Input: part model. Units: mm. Frame: model coordinates. A direction names the side the tool comes from. Give positions to 0.01 mm unless a question says otherwise; leave off trailing zeros. Loops run counter-clockwise (first coordinate to the right, second up) from the corner with the lowest first, then second, coordinate; pieces in that order, holes last.
from build123d import *

# Parameters (mm, degrees)
SKETCH1_W           = 22
SKETCH1_H           = 4.5
BOSS_EXTRUDE1_DEPTH = 1
SKETCH2_W           = 4.5
SKETCH2_H           = 4.5
BOSS_EXTRUDE2_DEPTH = 5
FILLET1_R           = 0.5


with BuildPart() as part:
    # Sketch1 → Boss-Extrude1 (new body)
    with BuildSketch(Plane(origin=(0, 0, 0), x_dir=(1, 0, 0), z_dir=(0, 1, 0))):
        Rectangle(SKETCH1_W, SKETCH1_H)
    extrude(amount=BOSS_EXTRUDE1_DEPTH)

    # Sketch2 → Boss-Extrude2 (add)
    with BuildSketch(Plane(origin=(0, 1, 0), x_dir=(1, 0, 0), z_dir=(0, 1, 0))):
        with Locations((-8.75, 0)):
            Rectangle(SKETCH2_W, SKETCH2_H)
        with Locations((8.75, 0)):
            Rectangle(SKETCH2_W, SKETCH2_H)
    extrude(amount=BOSS_EXTRUDE2_DEPTH)

    # Fillet1
    fillet1_edges = [part.edges().sort_by_distance(p)[0] for p in [
        (8.75, 6, -2.25),
        (11, 6, 0),
        (8.75, 6, 2.25),
        (6.5, 6, 0),
        (-6.5, 6, 0),
        (-8.75, 6, 2.25),
        (-11, 6, 0),
        (-8.75, 6, -2.25),
    ]]
    fillet(fillet1_edges, radius=FILLET1_R)


solid = part.part
(1) Cut plane A-A (y = 2.15). Return the cut outline in (x, z).
Values follow:
outline: (-11, -2.25) - (-6.5, -2.25) - (-6.5, 2.25) - (-11, 2.25) - close; (6.5, -2.25) - (11, -2.25) - (11, 2.25) - (6.5, 2.25) - close
(2) Cut plane B-B (z = 0.65). Return the cut outline in (x, y), and give its area (3 significant figures).
Values follow:
outline: (-11, 0) - (11, 0) - (11, 5.5) arc R0.5 ccw to (10.5, 6) - (7, 6) arc R0.5 ccw to (6.5, 5.5) - (6.5, 1) - (-6.5, 1) - (-6.5, 5.5) arc R0.5 ccw to (-7, 6) - (-10.5, 6) arc R0.5 ccw to (-11, 5.5) - close
area: 66.8 mm2
(3) Cut plane C-C (x = -5.5). Return the cut outline in (y, z).
Values follow:
outline: (0, -2.25) - (1, -2.25) - (1, 2.25) - (0, 2.25) - close
(4) Pin query (flat end, axial travel): pin 1 Ø1.3 at (x, z) = (0, 1) entering from +Y. Return the tip coordinate at first contact, or that it passes through.
Values follow:
pin 1: stops at y = 1
(5) Mould query, pull axis X, two halves, no side actions, for faces 3 (the flat face through (-6.5, 3, 0)), 4 (the flat face through (11, 3, 0)), 5 (the flat face through (-11, 3, 0)), 6 (the flat face through (-0.2, 0.3, 2.25)). Classes: +X half, -X half, draft (parallel to the pull), parting line (faces both ways), or undercut.
Values follow:
face 3: undercut
face 4: +X half
face 5: -X half
face 6: draft
(6) Reachability of faces 1 (the flat face through (-0.2, 0.3, -2.25)), 2 (the flat face through (0, 1, 0)) from +Z, -Z, +X, -X, +Y, -Y: full face, straight path, thin tool, end or side. Return the list, or none.
Values follow:
face 1: -Z, +X, -X, +Y, -Y
face 2: +Z, -Z, +Y
(7) Ray query, probe 1 along X at (y, z) = (5.1, -0.75); probe 2 along Y at (x, z) = (-5.75, 1.1); probe 3 along X at (y, z) = (5.75, -1.05). Return the intervals inside material, ascending.
Values follow:
probe 1: x = -11 to -6.5, 6.5 to 11
probe 2: y = 0 to 1
probe 3: x = -10.93 to -6.57, 6.57 to 10.93
